```python
from build123d import *

# Parameters (mm, degrees)
SKETCH_1_W           = 22.333333334
SKETCH_1_H           = 10
EXTRUDE_1_DEPTH      = 30
SKETCH_4_W           = 1.083333334
SKETCH_4_H           = 30
CUT_EXTRUDE_1_DEPTH  = 30
SKETCH_3_R           = 2.25
CUT_EXTRUDE_2_DEPTH  = 15
SKETCH_5_OUTSIDE_W   = 30.87
SKETCH_5_OUTSIDE_H   = 19.62
SKETCH_5_OUTSIDE_W_2 = 18.7
SKETCH_5_OUTSIDE_H_2 = 8.315719237
CUT_EXTRUDE_3_DEPTH  = 30
SKETCH_10_W          = 18.7
SKETCH_10_H          = 8.304405234
EXTRUDE_2_DEPTH      = 18
SKETCH_11_W          = 20
SKETCH_11_H          = 2.687046706
CUT_EXTRUDE_5_DEPTH  = 36.702801011
CUT_EXTRUDE_6_DEPTH  = 32.955789688
SKETCH_13_W          = 18.7
SKETCH_13_H          = 5
EXTRUDE_3_DEPTH      = 5.617358528
SKETCH_15_W          = 18.7
SKETCH_15_H          = 25
CUT_EXTRUDE_7_DEPTH  = 33.535840608
SKETCH_18_W          = 28
SKETCH_18_H          = 8.304405234
EXTRUDE_5_DEPTH      = 0.85
SKETCH_20_W          = 5
SKETCH_20_H          = 28
EXTRUDE_6_DEPTH      = 52
EXTRUDE_7_DEPTH      = 5
SKETCH_22_R          = 10
CUT_EXTRUDE_8_DEPTH  = 63.24117166
EXTRUDE_8_DEPTH      = 20
SKETCH_30_W          = 5
SKETCH_30_H          = 20
CUT_EXTRUDE_10_DEPTH = 20.81
EXTRUDE_9_DEPTH      = 15
EXTRUDE_9_DEPTH_BACK = 20
SKETCH_31_W          = 20
SKETCH_31_H          = 3
SKETCH_32_R          = 2.55
CUT_EXTRUDE_11_DEPTH = 52.125105162
SKETCH_33_W          = 4.55
SKETCH_33_H          = 20
EXTRUDE_10_DEPTH     = 31.19
SKETCH_34_R          = 11.05
CUT_EXTRUDE_12_DEPTH = 10


with BuildPart() as part:
    # 草图1 → 凸台-拉伸1 (new body)
    with BuildSketch(Plane.XY):
        Rectangle(SKETCH_1_W, SKETCH_1_H)
    extrude(amount=EXTRUDE_1_DEPTH)

    # 草图4 → 切除-拉伸1 (cut)
    with BuildSketch(Plane.XZ.offset(5)):
        with Locations((-10.625, 15)):
            Rectangle(SKETCH_4_W, SKETCH_4_H)
    extrude(amount=-CUT_EXTRUDE_1_DEPTH, mode=Mode.SUBTRACT)

    # 草图3 → 切除-拉伸2 (cut)
    with BuildSketch(Plane.XY.offset(30)):
        with Locations((-4.883333333, -0.3)):
            Circle(SKETCH_3_R)
        with Locations((5.116666667, -0.3)):
            Circle(SKETCH_3_R)
    extrude(amount=-CUT_EXTRUDE_2_DEPTH, mode=Mode.SUBTRACT)

    # 草图5 outside → 切除-拉伸3 (cut)
    with BuildSketch(Plane.XY.offset(30)):
        with Locations((0.542, 0)):
            Rectangle(SKETCH_5_OUTSIDE_W, SKETCH_5_OUTSIDE_H)
        with Locations((0.116666667, -0.853454385)):
            Rectangle(SKETCH_5_OUTSIDE_W_2, SKETCH_5_OUTSIDE_H_2, mode=Mode.SUBTRACT)
    extrude(amount=-CUT_EXTRUDE_3_DEPTH, mode=Mode.SUBTRACT)

    # 草图10 → 凸台-拉伸2 (add)
    with BuildSketch(Plane(origin=(0, 0, 0), x_dir=(-1, 0, 0), z_dir=(0, 0, -1))):
        with Locations((-0.116666667, -0.847797383)):
            Rectangle(SKETCH_10_W, SKETCH_10_H)
    extrude(amount=EXTRUDE_2_DEPTH)

    # 草图11 → 切除-拉伸5 (cut, through all)
    with BuildSketch(Plane(origin=(9.466666667, 0, 0), x_dir=(0, 0, -1), z_dir=(1, 0, 0))):
        with Locations((8, -3.656476647)):
            Rectangle(SKETCH_11_W, SKETCH_11_H)
    extrude(amount=-CUT_EXTRUDE_5_DEPTH, mode=Mode.SUBTRACT)

    # 草图12 → 切除-拉伸6 (cut, through all)
    with BuildSketch(Plane.XZ.offset(2.312953294)):
        with BuildLine():
            ThreePointArc((-2.185193673, -12.99813966), (-4.733333333, -10.45), (-7.281472993, -12.99813966))
            Line((-7.281472993, -12.99813966), (-2.185193673, -12.99813966))
        make_face()
        with BuildLine():
            Line((-2.185193673, -12.99813966), (-7.281472993, -12.99813966))
            ThreePointArc((-7.281472993, -12.99813966), (-4.733333333, -15.54627932), (-2.185193673, -12.99813966))
        make_face()
        with BuildLine():
            ThreePointArc((7.514806327, -12.99813966), (4.966666667, -10.45), (2.418527007, -12.99813966))
            Line((2.418527007, -12.99813966), (7.514806327, -12.99813966))
        make_face()
        with BuildLine():
            Line((7.514806327, -12.99813966), (2.418527007, -12.99813966))
            ThreePointArc((2.418527007, -12.99813966), (4.966666667, -15.54627932), (7.514806327, -12.99813966))
        make_face()
    extrude(amount=-CUT_EXTRUDE_6_DEPTH, mode=Mode.SUBTRACT)

    # 草图13 → 凸台-拉伸3 (add)
    with BuildSketch(Plane(origin=(0, 3.304405234, 0), x_dir=(1, 0, 0), z_dir=(0, 1, 0))):
        with Locations((0.116666667, 20.5)):
            Rectangle(SKETCH_13_W, SKETCH_13_H)
    extrude(amount=-EXTRUDE_3_DEPTH)

    # 草图15 → 切除-拉伸7 (cut, through all)
    with BuildSketch(Plane.XZ.offset(5)):
        with Locations((0.116666667, -10.5)):
            Rectangle(SKETCH_15_W, SKETCH_15_H)
    extrude(amount=-CUT_EXTRUDE_7_DEPTH, mode=Mode.SUBTRACT)

    # 草图18 → 凸台-拉伸5 (add)
    with BuildSketch(Plane(origin=(9.466666667, 0, 0), x_dir=(0, 0, -1), z_dir=(1, 0, 0))):
        with Locations((-16, -0.847797383)):
            Rectangle(SKETCH_18_W, SKETCH_18_H)
    extrude(amount=EXTRUDE_5_DEPTH)

    # 草图20 → 凸台-拉伸6 (add)
    with BuildSketch(Plane(origin=(0, 3.304405234, 0), x_dir=(1, 0, 0), z_dir=(0, 1, 0))):
        with Locations((12.816666667, -16)):
            Rectangle(SKETCH_20_W, SKETCH_20_H)
    extrude(amount=-EXTRUDE_6_DEPTH)

    # 草图23 → 凸台-拉伸7 (add)
    with BuildSketch(Plane(origin=(0, 0, 2), x_dir=(-1, 0, 0), z_dir=(0, 0, -1))):
        Polygon((9.233333333, 3.304405234), (-15.316666667, 3.304405234), (-15.316666667, -48.695594766), (-10.316666667, -48.695594766), (-10.316666667, -5), (9.233333333, -5), align=None)
    extrude(amount=EXTRUDE_7_DEPTH)

    # 草图22 → 切除-拉伸8 (cut, through all)
    with BuildSketch(Plane(origin=(15.316666667, 0, 0), x_dir=(0, 0, -1), z_dir=(1, 0, 0))):
        with Locations((-10.741872617, -35.1)):
            Circle(SKETCH_22_R)
    extrude(amount=-CUT_EXTRUDE_8_DEPTH, mode=Mode.SUBTRACT)

    # 草图24 → 凸台-拉伸8 (add)
    with BuildSketch(Plane(origin=(0, 0, -3), x_dir=(-1, 0, 0), z_dir=(0, 0, -1))):
        Polygon((-10.316666667, -5), (-10.316666667, 3.304405234), (-15.316666667, 3.304405234), (-15.316666667, -48.695594766), (-10.316666667, -48.695594766), align=None)
    extrude(amount=EXTRUDE_8_DEPTH)

    # 草图30 → 切除-拉伸10 (cut)
    with BuildSketch(Plane.XZ.offset(48.695594766)):
        with Locations((12.816666667, -13)):
            Rectangle(SKETCH_30_W, SKETCH_30_H)
    extrude(amount=-CUT_EXTRUDE_10_DEPTH, mode=Mode.SUBTRACT)

    # 草图31 → 凸台-拉伸9 (add, two sides: drawn at the far end of the back side and taken through both)
    with BuildSketch(Plane(origin=(15.316666667, 0, 0), x_dir=(0, 0, -1), z_dir=(1, 0, 0)).offset(-EXTRUDE_9_DEPTH_BACK)):
        with Locations((13, -26.385594766)):
            Rectangle(SKETCH_31_W, SKETCH_31_H)
    extrude(amount=EXTRUDE_9_DEPTH + EXTRUDE_9_DEPTH_BACK)

    # 草图32 → 切除-拉伸11 (cut, through all)
    with BuildSketch(Plane(origin=(0, -24.885594766, 0), x_dir=(1, 0, 0), z_dir=(0, 1, 0))):
        with Locations(Location((3.000831302, 13, 0), (0, 0, 270))):
            Circle(SKETCH_32_R)
        with Locations(Location((22.632502032, 13, 0), (0, 0, 270))):
            Circle(SKETCH_32_R)
    extrude(amount=-CUT_EXTRUDE_11_DEPTH, mode=Mode.SUBTRACT)

    # 草图33 → 凸台-拉伸10 (add)
    with BuildSketch(Plane(origin=(0, 3.304405234, 0), x_dir=(1, 0, 0), z_dir=(0, 1, 0))):
        with Locations((-6.958333333, 13)):
            Rectangle(SKETCH_33_W, SKETCH_33_H)
    extrude(amount=-EXTRUDE_10_DEPTH)

    # 草图34 → 切除-拉伸12 (cut)
    with BuildSketch(Plane(origin=(15.316666667, 0, 0), x_dir=(0, 0, -1), z_dir=(1, 0, 0))):
        with Locations((-10.741872617, -35.1)):
            Circle(SKETCH_34_R)
    extrude(amount=-CUT_EXTRUDE_12_DEPTH, mode=Mode.SUBTRACT)


solid = part.part
```
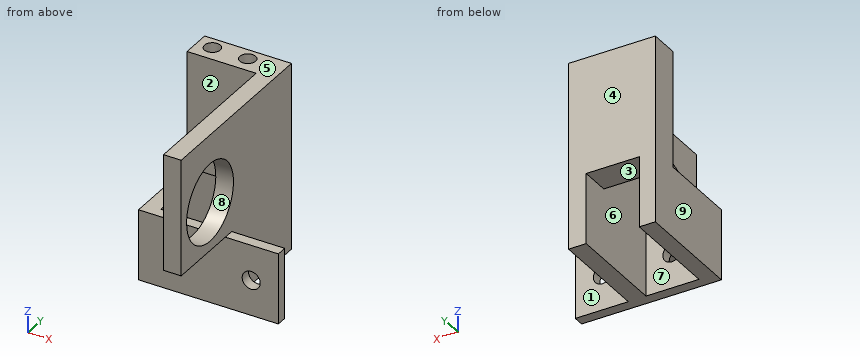
For this review, take the finished solid that the model builds, in its own axes (mm). Face numbers are marked on the shaded views. A direction names the side the tool comes from. Coordinates: 2 decimals unless noted, no trailing zeros. Loops run counter-clockwise (first coordinate to the right, second up) from the corner with the lowest first, then second, coordinate; pieces in that order, holes last. Notation, with made-up numbers: (84.25, 81.5) - (93.25, 81.5) arc R18 cw to (93.25, 97.5) - close; hole circle Ø6 at (75.25, -33.75). An arc over 180 degrees is marked (long way). Use one line per item in the form item = value. Start each with the question number.
1) To check wall thickness, follow probe 1 along X at (y, z) = (-26.1, -13); probe 2 along X at (y, z) = (-19.5, -5.5); probe 3 along Y at (x, z) = (-6.5, -3.5). State the ranges of each line that lie inside material, in increasing order. Write a range as from..to.
2) Take a section at B-B (z = -13). State the section outline as (x, y) points, plus the area to 3 significant figures.
3) For pin 1 (1.5 mm diameter, centred on x = 4.5, z = -0.5, fed in from -Y); pin 2 (4 mm diameter, centred on x = -4.88, y = -0.3, fed in from +Z); pin 3 (3.5 mm diameter, centred on x = 22, y = -27, fed in from +Z), all flat-tipped, find the tip position at first contact; note any pin that passes through.
4) For the marked faces 1, 2, 3, 4 and 5, list the 3-axis set-ups (+Z, -Z, +X, -X, +Y, -Y) from which the entire face can be reached by the end or side of a thin tool; tool diameter is ignored.
5) Take a section at A-A (y = -35.1). State the section outline as (x, z) points.
6) Draft analysis for pull direction X (two halves, no side actions). For the marked faces 6, 7, 8 and 9, state which applies: released by +X, released by -X, zero draft, split by the parting line, or undercut.
7) Take a section at C-C (z = 20.5). State the section outline as (x, y) points, plus the area to 3 significant figures.
8) Take a section at D-D (x = 6.5). State the section outline as (y, z) points, plus the area to 3 significant figures.
From the geometry:
q1.probe_1 = -9.23..0.45, 5.55..20.08, 25.18..30.32
q1.probe_2 = -9.23..-4.68, 10.32..15.32
q1.probe_3 = -27.89..3.3
q2.outline = (-9.23, -27.89) - (0.45, -27.89) - (0.45, -24.89) - (-4.68, -24.89) - (-4.68, 3.3) - (-9.23, 3.3) - close; (5.55, -27.89) - (20.08, -27.89) - (20.08, -24.89) - (15.32, -24.89) - (15.32, 3.3) - (10.32, 3.3) - (10.32, -24.89) - (5.55, -24.89) - close; (25.18, -27.89) - (30.32, -27.89) - (30.32, -24.89) - (25.18, -24.89) - close
q2.area = 357 mm2
q3.pin_1 = -5
q3.pin_2 = 15
q3.pin_3 = -3
q4.face_1 = +Z, -Z, +X, +Y
q4.face_2 = +Z, -X, -Y
q4.face_3 = -Z, +Y
q4.face_4 = +Z, -Z, +X, -X, +Y
q4.face_5 = +Z, +X, -X, +Y, -Y
q5.outline = (10.32, -3) - (15.32, -3) - (15.32, -0.31) - (10.32, -0.31) - close; (10.32, 21.79) - (15.32, 21.79) - (15.32, 30) - (10.32, 30) - close
q6.face_6 = undercut
q6.face_7 = undercut
q6.face_8 = zero draft
q6.face_9 = released by -X
q7.outline = (-9.23, -5) - (10.32, -5) - (10.32, -29.92) - (15.32, -29.92) - (15.32, 3.3) - (-9.23, 3.3) - close; (10.32, -48.7) - (15.32, -48.7) - (15.32, -40.28) - (10.32, -40.28) - close; hole circle Ø4.5 at (-4.88, -0.3); hole circle Ø4.5 at (5.12, -0.3)
q7.area = 339 mm2
q8.outline = (-27.89, -23) - (-24.89, -23) - (-24.89, -3) - (-27.89, -3) - close; (-5, -3) - (3.3, -3) - (3.3, 30) - (1.47, 30) - (1.47, 15) - (-2.07, 15) - (-2.07, 30) - (-5, 30) - close
q8.area = 281 mm2
